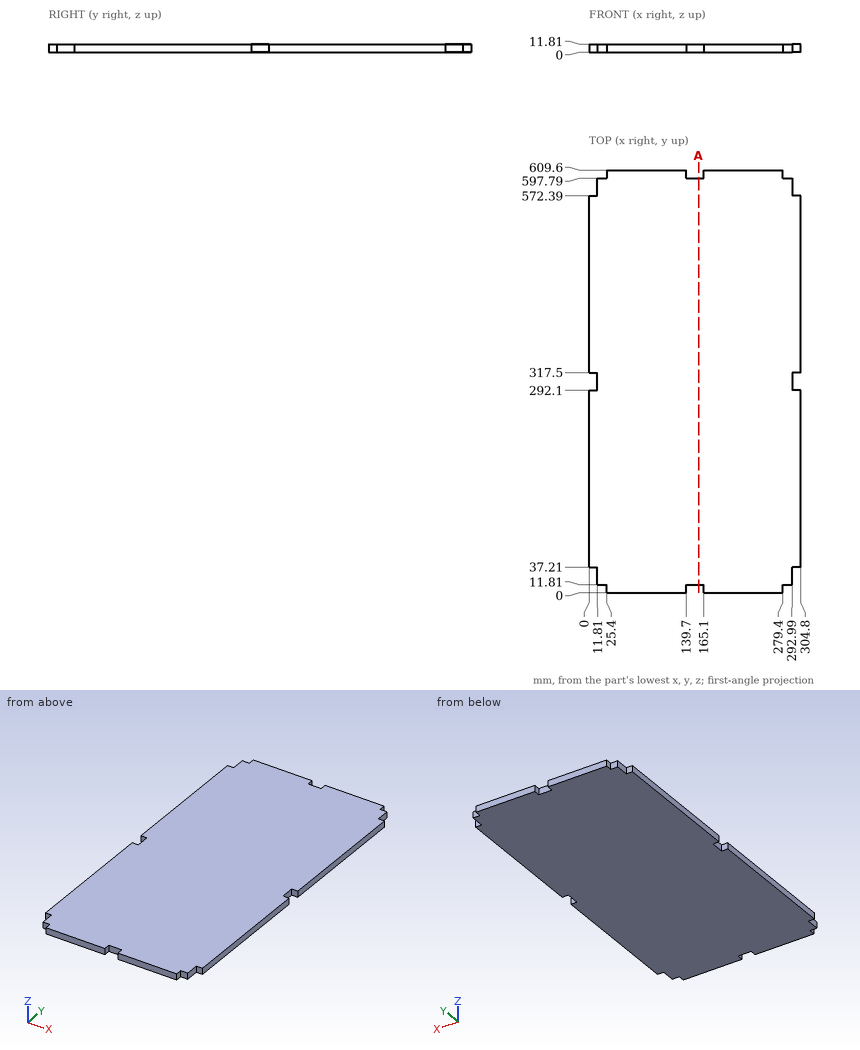
Study the drawing (mm; zero at the part's minimum x, y, z) and answer. Round coordinates to 2 decimals unless told otherwise and drop trailing zeros. Loops run counter-clockwise (first coordinate to the right, second up) from the corner with the lowest first, then second, coordinate; pieces in that order, holes last. Notation, with made-up numbers: (46, 46) -> (55, 46) arc R13 ccw to (55, 68) -> close; hole circle Ø5 at (-1.75, 89). An arc over 180 degrees is marked (long way). One line per item, written item: value.
1) Consider L1, parallel to Y at x = 142, z = 4.75; L2, parallel to X at y = 300, z = 4.75. Determine where each line is inside the solid, lowest interval first. Write a range as [from, to].
Answer list:
L1: y = [11.81, 597.79]
L2: x = [11.81, 292.99]
2) A cutting plane is placed at A-A (x = 158). Determine the outline of the cut face in (y, z).
Answer list:
outline: (11.81, 0) -> (597.79, 0) -> (597.79, 11.81) -> (11.81, 11.81) -> close
3) Flat-ended cylindrical pins translate along their axes: P1, Ø3.5, axis at x = 21, z = 8, coming from the -Y side; P2, Ø6, axis at y = 3.5, z = 6.5, coming from the -X side; P3, Ø3.5, axis at x = 301.5, z = 6.5, coming from the -Y side. Find the tip coordinate at first contact, or state that the pin passes through.
Answer list:
P1: stops at y = 11.81
P2: stops at x = 25.4
P3: stops at y = 37.21
